Source: CAD feature listing. Evaluate the final solid. Frame: model axes, mm. Face numbers are marked on the shaded views. Give positions to 0.01 mm unless a question says otherwise; leave off trailing zeros. Write each loop counter-clockwise with the first axis right and the second up, starting at its lowest first coordinate (ties: lowest second). Pieces come first, ordered by that corner, then holes. Notation, with made-up numbers: (-34.75, 44) -> (-20.75, 44) arc R29 ccw to (-20.75, 66) -> close; hole circle Ø6 at (-22.5, -31). An arc over 180 degrees is marked (long way). Use a Markdown table: item, result. Add a question column.
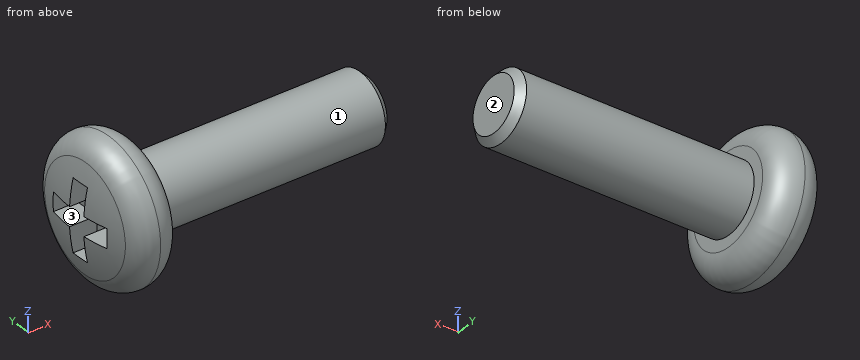
Autodesk Inventor part; units mm, degrees
ref_plane "РабПлоскость2" through (-12.3726, 0, 0) normal (1, 0, 0) x (0, 0, -1)
ref_plane "YZ Plane" through (0, 0, 0) normal (1, 0, 0) x (0, 1, 0)
ref_plane "XZ Plane" through (0, 0, 0) normal (0, 1, 0) x (-1, 0, 0)
sketch "Эскиз1" plane through (0, 0, 0) normal (0, 0, 1) x (1, 0, 0)
  line L0 (0, 0) -> (-12.3726, 0)
  arc A0 (-10, 1.9227) -> (-12, 2.2534) centre (-11.0273, 1.9227) ccw
  line L1 (-10, 1.9227) -> (-10, 1.45)
  line L2 (-10, 1.45) -> (0, 1.45)
  line L3 (0, 1.45) -> (0, 0)
  line L4 (-12.6724, 2.95) -> (-10.1128, 2.95)
  arc A1 (-12, 2.2534) -> (-12.3726, 0) centre (-5.3726, 0) ccw
  dimension "d0" = 2.9
  dimension "d1" = 5.9
  dimension "d2" = 2
  dimension "d3" = 10
  dimension "d4" = 7
revolve "Вращение1" add sketch "Эскиз1" angle 360 about axis through (0, 0, 0) along (-1, 0, 0)
chamfer "Фаска1" distance 0.3 angle 45 1 edges at (0, -1.45, 0)
ref_plane "РабПлоскость2" through (-12.3726, 0, 0) normal (1, 0, 0) x (0, 0, -1)
sketch "Эскиз2" plane through (-12.3726, 0, 0) normal (1, 0, 0) x (0, 0, -1)
  line L0 (-0.4, 1.5) -> (0.4, 1.5)
  line L1 (0.4, 1.5) -> (0.4, -1.5)
  line L2 (0.4, -1.5) -> (-0.4, -1.5)
  line L3 (-0.4, -1.5) -> (-0.4, 1.5)
  line L4 (-1.5, 0.4) -> (1.5, 0.4)
  line L5 (1.5, 0.4) -> (1.5, -0.4)
  line L6 (1.5, -0.4) -> (-1.5, -0.4)
  line L7 (-1.5, -0.4) -> (-1.5, 0.4)
  point P0 (0, 0)
  point P1 (0, 1.5)
  point P2 (0, 0.4)
  point P3 (-1.5, 0)
  point P4 (-0.4, 0)
  point P5 (0.4, 0.4)
  point P6 (-0.4, 0.4)
  point P7 (-0.4, -0.4)
  point P8 (0.4, -0.4)
  dimension "d10" = 0.8
  dimension "d11" = 3
extrude "Выдавливание1" cut sketch "Эскиз2" along normal blind 1.2
properties part number "Винт М3х19"
(1) Material intervals for L1, parallel to X at y = -0.2, z = -1.1; L2, parallel to Y at x = -2.75, z = 0; L3, parallel to X at y = 1.75, z = 1.7, sorted ascending.
(2) Cut plane A-A on x = -7.5. Return the cut outline in (y, z).
(3) Mould query, pull axis Z, two halves, no side actions, for the marked faces 1, 2 and 3. Classes: +Z half, -Z half, draft (parallel to the pull), parting line (faces both ways), or undercut.
(4) First-contact query: pin 1 Ø0.9 at (x, y) = (-11.5, 0) entering from +Z; pin 2 Ø0.6 at (x, y) = (-11.5, 1) entering from -Z; pin 3 Ø3 at (x, z) = (-9.5, -1) entering from -Y; pin 4 Ø1.5 at (y, z) = (0.5, 2) entering from +X. Flat tips, straight axial feed; report the tip coordinate or a pass-through.
Output:
| question | item | result |
|---|---|---|
| 1 | L1 | -11.17 to 0 |
| 1 | L2 | -1.45 to 1.45 |
| 1 | L3 | -11.92 to -10.14 |
| 2 | outline | circle Ø2.9 at (0, 0) |
| 3 | face 1 | parting line |
| 3 | face 2 | draft |
| 3 | face 3 | undercut |
| 4 | pin 1 | z = 2.95 |
| 4 | pin 2 | z = -2.81 |
| 4 | pin 3 | y = -2.91 |
| 4 | pin 4 | x = -0.16 |
